```python
from build123d import *

# Parameters (mm, degrees)
SKETCH1_W           = 112
SKETCH1_H           = 88.12
SKETCH1_R           = 21
SKETCH1_R_2         = 2.25
BOSS_EXTRUDE1_DEPTH = 3.5
SKETCH2_R           = 1.997849158
SKETCH2_R_2         = 1.997849136
SKETCH2_R_3         = 1.997849041
SKETCH2_R_4         = 1.99784915
CUT_EXTRUDE1_DEPTH  = 3.5


with BuildPart() as part:
    # Sketch1 → Boss-Extrude1 (new body)
    with BuildSketch(Plane.XY):
        Rectangle(SKETCH1_W, SKETCH1_H)
        Circle(SKETCH1_R, mode=Mode.SUBTRACT)
        with Locations((25, 0)):
            Circle(SKETCH1_R_2, mode=Mode.SUBTRACT)
        with Locations((23, 9.797958971)):
            Circle(SKETCH1_R_2, mode=Mode.SUBTRACT)
        with Locations((23, -9.797958971)):
            Circle(SKETCH1_R_2, mode=Mode.SUBTRACT)
        with Locations((-23, 9.797958971)):
            Circle(SKETCH1_R_2, mode=Mode.SUBTRACT)
        with Locations((-25, 0)):
            Circle(SKETCH1_R_2, mode=Mode.SUBTRACT)
        with Locations((-23, -9.797958971)):
            Circle(SKETCH1_R_2, mode=Mode.SUBTRACT)
    extrude(amount=BOSS_EXTRUDE1_DEPTH)

    # Sketch2 → Cut-Extrude1 (cut)
    with BuildSketch(Plane.XY.offset(3.5)):
        with Locations((-41.749999967, 11.002177996)):
            Circle(SKETCH2_R)
        with Locations((41.750000033, 38.997821996)):
            Circle(SKETCH2_R)
        with Locations((-41.749999967, 39.002177996)):
            Circle(SKETCH2_R)
        with Locations((41.750000033, 10.997821996)):
            Circle(SKETCH2_R)
        with Locations((41.75, -10.997822003)):
            Circle(SKETCH2_R_2)
        with Locations((41.75, -38.997822003)):
            Circle(SKETCH2_R_2)
        with Locations((-41.749999857, -38.997821959)):
            Circle(SKETCH2_R_3)
        with Locations((-41.749999952, -10.997822035)):
            Circle(SKETCH2_R_4)
    extrude(amount=-CUT_EXTRUDE1_DEPTH, mode=Mode.SUBTRACT)


solid = part.part
```
Check sheet for the modelled part. Datum: model origin and axes. Units: mm. Give positions to 0.01 mm unless a question says otherwise; leave off trailing zeros. Order: outer loops, then holes, each group sorted by start corner. A loop starts at its lowest first (then second) coordinate and runs counter-clockwise, first axis right, second up. Notation, with made-up numbers: M 87.5,-33.5 L 116.5,-33.5 A15 ccw 116.5,-18.5 Z; hole C -14,65.5 d9. An arc over 180 degrees is marked long. Answer in a Markdown table with one row per item. Add a question column.
Q1. Thickness scan on L1, parallel to Y at x = -41.75, z = 1.35; L2, parallel to Y at x = 25, z = 2.7; L3, parallel to Y at x = -23, z = 1.55. Record the ranges inside material, lowest first.
Q2. Sectioned sample at C-C, the plane x = -41.75. Record the boundary of the cut face in (y, z).
Q3. Gauge pin test, flat end, axial feed: pin 1 Ø2.5 at (x, y) = (-41.75, -39) entering from -Z. Record the tip position at first contact, or that the pin passes through.
Q4. Sectioned sample at A-A, the plane x = 0. Record the boundary of the cut face in (y, z), and give its area (3 significant figures).
Q5. Sectioned sample at B-B, the plane y = 0. Record the boundary of the cut face in (x, z).
Q6. Sectioned sample at D-D, the plane z = 1.9. Count the separate pieces of the cut face and the enclosed holes in it, and give its area (3 significant figures).
Q7. Release check for a two-part mould opening along Y. For faces 1 (the flat face through (-13, 20, 3.5)), 2 (the cylindrical face through (-40.7, 40.7, 1.8)), 3 (the flat face through (-1, 44.06, 2)) record: released by +Y, released by -Y, zero draft, split by the parting line, or undercut.
Verdict:
| question | item | result |
|---|---|---|
| 1 | L1 | -44.06 to -41, -37 to -13, -9 to 9, 13 to 37, 41 to 44.06 |
| 1 | L2 | -44.06 to -10.83, -8.77 to -2.25, 2.25 to 8.77, 10.83 to 44.06 |
| 1 | L3 | -44.06 to -12.05, -7.55 to -1.03, 1.03 to 7.55, 12.05 to 44.06 |
| 2 | outline | M -44.06,0 L -41,0 L -41,3.5 L -44.06,3.5 Z; M -37,0 L -13,0 L -13,3.5 L -37,3.5 Z; M -9,0 L 9,0 L 9,3.5 L -9,3.5 Z; M 13,0 L 37,0 L 37,3.5 L 13,3.5 Z; M 41,0 L 44.06,0 L 44.06,3.5 L 41,3.5 Z |
| 3 | pin 1 | through |
| 4 | outline | M -44.06,0 L -21,0 L -21,3.5 L -44.06,3.5 Z; M 21,0 L 44.06,0 L 44.06,3.5 L 21,3.5 Z |
| 4 | area | 161 mm² |
| 5 | outline | M -56,0 L -27.25,0 L -27.25,3.5 L -56,3.5 Z; M -22.75,0 L -21,0 L -21,3.5 L -22.75,3.5 Z; M 21,0 L 22.75,0 L 22.75,3.5 L 21,3.5 Z; M 27.25,0 L 56,0 L 56,3.5 L 27.25,3.5 Z |
| 6 | separate pieces | 1 |
| 6 | enclosed holes | 15 |
| 6 | area | 8,290 mm² |
| 7 | face 1 | zero draft |
| 7 | face 2 | undercut |
| 7 | face 3 | released by +Y |
